Autodesk Inventor part; units mm, degrees
ref_plane "YZ Plane" through (0, 0, 0) normal (1, 0, 0) x (0, 1, 0)
ref_plane "XZ Plane" through (0, 0, 0) normal (0, 1, 0) x (-1, 0, 0)
ref_plane "XY Plane" through (0, 0, 0) normal (0, 0, 1) x (1, 0, 0)
sketch "Sketch2" plane through (0, 0, 0) normal (0, 1, 0) x (-1, 0, 0)
  line L0 (-3.48, 2.7) -> (3.48, 2.7)
  arc A0 (3.48, 2.7) -> (5.28, 4.5) centre (3.48, 4.5) ccw
  line L1 (5.28, 4.5) -> (5.28, 7.38)
  line L2 (5.28, 7.38) -> (8, 7.38)
  line L3 (8, 7.38) -> (8, 2.62)
  line L4 (8, 2.62) -> (10.62, 0)
  line L5 (10.62, 0) -> (4, -6.62)
  line L6 (4, -6.62) -> (-4, -6.62)
  line L7 (-4, -6.62) -> (-10.62, 0)
  line L8 (-10.62, 0) -> (-8, 2.62)
  line L9 (-8, 2.62) -> (-8, 7.38)
  line L10 (-8, 7.38) -> (-5.28, 7.38)
  line L11 (-5.28, 7.38) -> (-5.28, 4.5)
  arc A1 (-5.28, 4.5) -> (-3.48, 2.7) centre (-3.48, 4.5) ccw
  point P0 (0, 0)
  point P1 (0, 2.7)
  point P2 (0, -6.62)
  dimension "d0" = 1.8
  dimension "d1" = 4.68
  dimension "d2" = 2.72
  dimension "d3" = 10.56
  dimension "d4" = 4.76
  dimension "d5" = 9.32
  dimension "d6" = 8
extrude "Extrusion1" add sketch "Sketch2" along normal mid plane 5.2
fillet "Fillet1" radius 0.6 6 edges at (-8, 0, 7.38) (-5.28, 0, 7.38) (5.28, 0, 7.38) (8, 0, 7.38) (10.62, 0, 0) (-10.62, 0, 0)
chamfer "Chamfer1" distance 0.12 angle 45 20 edges at (-8, 2.6, 4.7) (-7.8243, 2.6, 7.2043) (-6.64, 2.6, 7.38) (-5.4557, 2.6, 7.2043) (-5.28, 2.6, 5.64) (-4.7528, 2.6, 3.2272) (0, 2.6, 2.7) (4.7528, 2.6, 3.2272) (5.28, 2.6, 5.64) (5.4557, 2.6, 7.2043) (6.64, 2.6, 7.38) (7.8243, 2.6, 7.2043) (8, 2.6, 4.7) (-9.0979, 2.6, 1.5221) (-10.3715, 2.6, 0) (-7.0979, 2.6, -3.5221) (0, 2.6, -6.62) (7.0979, 2.6, -3.5221) (10.3715, 2.6, 0) (9.0979, 2.6, 1.5221)
equation "\"d6\" = lu"
properties part number "99147-LtBluishGray" material "ABS Plastic"
The model under review builds one solid part; all positions refer to its coordinate system, in mm. A direction names the side the tool comes from. Give positions to 0.01 mm unless a question says otherwise; leave off trailing zeros. Write each loop counter-clockwise with the first axis right and the second up, starting at its lowest first coordinate (ties: lowest second). Pieces come first, ordered by that corner, then holes. Notation, with made-up numbers: M -10.5,-3.5 L -5.5,-3.5 A31 ccw -5.5,34.5 Z; hole C 43.5,39.25 d8. An arc over 180 degrees is marked long. Write each question's results on one line, items separated by ' | '. Start each with the question number.
1. We need section C-C (z = 1.5). Write out the cut boundary in (x, y).
2. Mouldability with a two-part tool opening along X and no side actions: class faces 4 (the flat face through (7.05, -0.1, -3.57)), 5 (the flat face through (0, 0, -6.62)), 6 (the cylindrical face through (4.739, -0.096, 3.213)) as released by +X, released by -X, zero draft, split by the parting line, or undercut.
3. For faces 1 (the flat face through (8, 0, 5)), 2 (the flat face through (0, -2.6, -1)), 3 (the cylindrical face through (-4.767, -0.096, 3.241)), list the 3-axis set-ups (+Z, -Z, +X, -X, +Y, -Y) from which the entire face can be reached by the end or side of a thin tool; tool diameter is ignored.
4. We need section A-A (y = -1.85). Write out the cut boundary in (x, z), and give its area (3 significant figures).
5. Insertion check: pin 1 Ø2 at (y, z) = (-1, 3) entering from -X; pin 2 Ø1.5 at (x, y) = (1, 0.5) entering from +Z; pin 3 Ø1.5 at (y, z) = (0, 4) entering from -X. Each pin has a flat end and moves straight along its axis. Give the tip position at first contact, or say it passes through.
6. For probe 1 along Z at (x, y) = (-2.75, 0.35); probe 2 along X at (y, z) = (2.3, 4); probe 3 along Z at (x, y) = (-9.5, 0.1), list the stretches that pass through material, from the lowest coordinate up. Write a range as [from, to].
7. We need section B-B (x = -1). Write out the cut boundary in (y, z).
Results found:
1) outline: M -9.12,-2.6 L 9.12,-2.6 L 9.12,2.48 L 8.95,2.6 L -8.95,2.6 L -9.12,2.48 Z
2) face 4: released by +X | face 5: zero draft | face 6: undercut
3) face 1: +Z, +X, +Y, -Y | face 2: +Z, -Z, +X, -X, -Y | face 3: +Z, +Y, -Y
4) outline: M -10.2,-0.42 L -4,-6.62 L 4,-6.62 L 10.2,-0.42 A0.6 ccw 10.2,0.42 L 8,2.62 L 8,6.78 A0.6 ccw 7.4,7.38 L 5.88,7.38 A0.6 ccw 5.28,6.78 L 5.28,4.5 A1.8 cw 3.48,2.7 L -3.48,2.7 A1.8 cw -5.28,4.5 L -5.28,6.78 A0.6 ccw -5.88,7.38 L -7.4,7.38 A0.6 ccw -8,6.78 L -8,2.62 L -10.2,0.42 A0.6 ccw Z | area: 173 mm^2
5) pin 1: stops at x = -8.62 | pin 2: stops at z = 2.7 | pin 3: stops at x = -8
6) probe 1: z = [-6.62, 2.7] | probe 2: x = [-8, -5.21], [5.21, 8] | probe 3: z = [-1.12, 1.12]
7) outline: M -2.6,-6.62 L 2.48,-6.62 L 2.6,-6.5 L 2.6,2.58 L 2.48,2.7 L -2.6,2.7 Z
